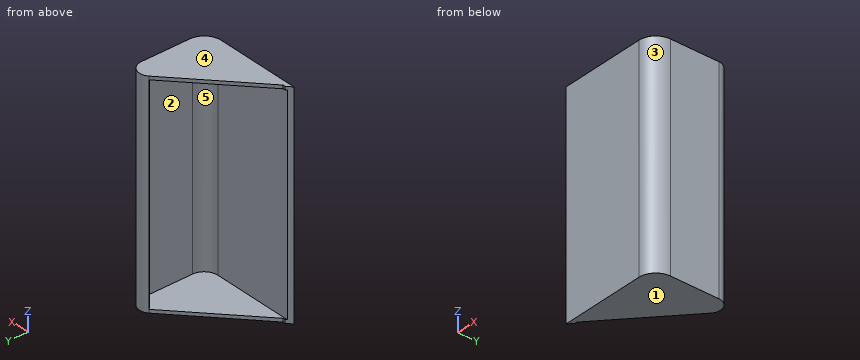
from build123d import *

# Parameters (mm, degrees)
BOSS_EXTRUDE1_DEPTH = 1900
SHELL1_START        = 30
SHELL1_DEPTH        = 1840
CUT_EXTRUDE1_DEPTH  = 2209.790719691


# Read off the part's stored shape, not the designer's step: Shell1
with BuildPart() as part:
    # Sketch2 → Boss-Extrude1 (new body)
    with BuildSketch(Plane.XY):
        with BuildLine():
            Line((0, 0), (750, 0))
            ThreePointArc((750, 0), (856.066017178, 43.933982822), (900, 150))
            Line((900, 150), (900, 577.315615791))
            ThreePointArc((900, 577.315615791), (840.965605157, 668.539621372), (733.563616117, 652.05654766))
            Line((733.563616117, 652.05654766), (0, 0))
        make_face()
    extrude(amount=BOSS_EXTRUDE1_DEPTH)

    # Shell1 outline → Shell1 (cut)
    with BuildSketch(Plane.XY.offset(SHELL1_START)):
        with BuildLine():
            Line((753.494531282, 629.634268099), (733.563616117, 652.05654766))
            Line((733.563616117, 652.05654766), (33.75, 30))
            Line((33.75, 30), (750, 30))
            ThreePointArc((750, 30), (834.852813742, 65.147186258), (870, 150))
            Line((870, 150), (870, 577.315615791))
            ThreePointArc((870, 577.315615791), (828.67592361, 641.172419698), (753.494531282, 629.634268099))
        make_face()
    extrude(amount=SHELL1_DEPTH, mode=Mode.SUBTRACT)

    # Sketch3 → Cut-Extrude1 (cut, through all)
    with BuildSketch(Plane.XY.offset(1900)):
        Polygon((45, 40), (65, 40), (733.563616117, 652.05654766), align=None)
    extrude(amount=-CUT_EXTRUDE1_DEPTH, mode=Mode.SUBTRACT)


solid = part.part
Input: part model. Units: mm. Frame: model coordinates. Face numbers are marked on the shaded views. A direction names the side the tool comes from. Give positions to 0.01 mm unless a question says otherwise; leave off trailing zeros. Order: outer loops, then holes, each group sorted by start corner. A loop starts at its lowest first (then second) coordinate and runs counter-clockwise, first axis right, second up. Notation, with made-up numbers: M 82,-28 L 132,-28 A22 cw 132,-12 Z; hole C -4,43.25 d11. An arc over 180 degrees is marked long. Answer as a JSON object with one key per item and string values.
1. Cut plane D-D, the plane y = 325. Output: boundary loops of the cut face in (x, z), and give its area (3 significant figures).
Result sheet:
{"outline": "M 376.31,0 L 900,0 L 900,1900 L 376.31,1900 L 376.31,1870 L 870,1870 L 870,30 L 376.31,30 Z", "area": "86,600 mm²"}
2. Cut plane A-A, the plane x = 796. Output: boundary loops of the cut face in (y, z), and give its area (3 significant figures).
Result sheet:
{"outline": "M 7.23,0 L 677.24,0 L 677.24,1900 L 7.23,1900 Z; hole M 39.17,30 L 647.2,30 L 647.2,1870 L 39.17,1870 Z", "area": "154,000 mm²"}
3. Ray query, line 1 (Z direction, x = 669, y = 177.5); line 2 (X direction, y = 563, z = 626); line 3 (X direction, y = 633.5, z = 87.5). Return the intervals inside material, ascending. Write a range as [from, to].
Result sheet:
{"line 1": "[0, 30], [1870, 1900]", "line 2": "[870, 900]", "line 3": "[750.06, 758.25], [841.75, 882.72]"}
4. Cut plane C-C, the plane x = 499.5. Output: boundary loops of the cut face in (y, z), and give its area (3 significant figures).
Result sheet:
{"outline": "M 0,0 L 437.78,0 L 437.78,30 L 30,30 L 30,1870 L 437.78,1870 L 437.78,1900 L 0,1900 Z", "area": "81,500 mm²"}
5. Pull-direction query (Z, two-part tool) for the marked faces 3, 4 and 5; classes: +Z half, -Z half, draft (parallel to the pull), parting line (faces both ways), or undercut.
Result sheet:
{"face 3": "draft", "face 4": "+Z half", "face 5": "undercut"}
6. First-contact query: P1, Ø10, axis at y = 142.5, z = 1124.5, coming from the +X side; P2, Ø5, axis at y = 436, z = 1478, coming from the -X side; P3, Ø5, axis at x = 244, z = 1489, coming from the +Y side. Flat tips, straight axial feed; report the tip coordinate or a pass-through.
Result sheet:
{"P1": "x = 899.98", "P2": "x = 870", "P3": "y = 30"}
7. Reachability of the marked faces 1 and 2 from +Z, -Z, +X, -X, +Y, -Y: full face, straight path, thin tool, end or side. Return the list, or none.
Result sheet:
{"face 1": "-Z, +X, -X, +Y, -Y", "face 2": "-X"}
8. Cut plane B-B, the plane z = 566.5. Output: boundary loops of the cut face in (x, y).
Result sheet:
{"outline": "M 0,0 L 750,0 A150 ccw 900,150 L 900,577.32 A100 ccw 733.56,652.06 L 753.49,629.63 A70 cw 870,577.32 L 870,150 A120 cw 750,30 L 33.75,30 Z"}
